```python
from build123d import *

# Parameters (mm, degrees)
SKETCH2_R                = 5
BOSS_EXTRUDE1_DEPTH      = 10
BOSS_EXTRUDE2_DEPTH      = 70
BOSS_EXTRUDE2_DEPTH_BACK = 20
SKETCH2_3_W              = 100
SKETCH2_3_H              = 10
SKETCH3_R                = 5
CUT_EXTRUDE1_DEPTH       = 5
FILLET1_R                = 2


with BuildPart() as part:
    # Sketch2 → Boss-Extrude1 (new body)
    with BuildSketch(Plane(origin=(0, 0, 0), x_dir=(0, 0, -1), z_dir=(1, 0, 0))):
        with BuildLine():
            Line((-8.38684039, 61.382374771), (-45, 5))
            Line((-45, 5), (45, 5))
            Line((45, 5), (8.38684039, 61.382374771))
            ThreePointArc((8.38684039, 61.382374771), (0, 65.936191862), (-8.38684039, 61.382374771))
        make_face()
        with Locations((0, 55.936191862)):
            Circle(SKETCH2_R, mode=Mode.SUBTRACT)
    extrude(amount=BOSS_EXTRUDE1_DEPTH)

    # Sketch2_3 → Boss-Extrude2 (add, two sides: drawn at the far end of the back side and taken through both)
    with BuildSketch(Plane(origin=(0, 0, 0), x_dir=(0, 0, -1), z_dir=(1, 0, 0)).offset(-BOSS_EXTRUDE2_DEPTH_BACK)):
        Rectangle(SKETCH2_3_W, SKETCH2_3_H)
    extrude(amount=BOSS_EXTRUDE2_DEPTH + BOSS_EXTRUDE2_DEPTH_BACK)

    # Sketch3 → Cut-Extrude1 (cut, symmetric)
    with BuildSketch(Plane(origin=(0, 0, 0), x_dir=(1, 0, 0), z_dir=(0, 1, 0))):
        with Locations(Location((60, 40, 0), (0, 0, 270))):
            Circle(SKETCH3_R)
        with Locations(Location((60, -40, 0), (0, 0, 270))):
            Circle(SKETCH3_R)
    extrude(amount=CUT_EXTRUDE1_DEPTH, both=True, mode=Mode.SUBTRACT)

    # Fillet1
    fillet1_edges = [part.edges().sort_by_distance(p)[0] for p in [
        (5, 5, -45),
        (5, 5, 45),
    ]]
    fillet(fillet1_edges, radius=FILLET1_R)


solid = part.part
```
Geometry check sheet. Reference: the model listing, model coordinates, mm. A direction names the side the tool comes from. Round coordinates to 2 decimals unless told otherwise and drop trailing zeros. Order: outer loops, then holes, each group sorted by start corner. A loop starts at its lowest first (then second) coordinate and runs counter-clockwise, first axis right, second up. Notation, with made-up numbers: M 76,-38.75 L 110,-38.75 A23 cw 110,0.25 Z; hole C 73,84.5 d4. An arc over 180 degrees is marked long. Write item = value, one per line.
Q1. Section check B-B (z = 0). Enter the section's corners in (x, y).
Answer block:
outline = M -20,-5 L 70,-5 L 70,5 L 10,5 L 10,50.94 L 0,50.94 L 0,5 L -20,5 Z; M 0,60.94 L 10,60.94 L 10,65.94 L 0,65.94 Z
Q2. Section check C-C (y = 57.5). Enter the section's corners in (x, z).
Answer block:
outline = M 0,-10.91 L 10,-10.91 L 10,-4.75 L 0,-4.75 Z; M 0,4.75 L 10,4.75 L 10,10.91 L 0,10.91 Z
Q3. Scan lines: line 1 (Y direction, x = 5.5, z = 0); line 2 (Z direction, x = 59, y = 1.5); line 3 (Y direction, x = 50, z = -27.5). Record each from-to range of solid material in increasing order.
Answer block:
line_1 = -5 to 50.94, 60.94 to 65.94
line_2 = -50 to -44.9, -35.1 to 35.1, 44.9 to 50
line_3 = -5 to 5
Q4. Section check A-A (x = 60). Enter the section's corners in (y, z).
Answer block:
outline = M -5,-50 L 5,-50 L 5,-45 L -5,-45 Z; M -5,-35 L 5,-35 L 5,35 L -5,35 Z; M -5,45 L 5,45 L 5,50 L -5,50 Z
Q5. Set-up check for faces 4 (the flat face through (0, 29, 1)), 5 (the flat face through (10, 29, 1)), 6 (the flat face through (70, 0, 1)): record each of +Z, -Z, +X, -X, +Y, -Y from which the full face is reachable in a straight line by a thin tool's end or side.
Answer block:
face_4 = +Z, -Z, -X, +Y
face_5 = +Z, -Z, +X, +Y
face_6 = +Z, -Z, +X, +Y, -Y
Q6. Section check D-D (x = 8). Enter the section's corners in (y, z), plus the area to 3 significant figures.
Answer block:
outline = M -5,-50 L 5,-50 L 5,-46.09 A2 cw 5.91,-44.41 L 61.38,-8.39 A10 ccw 61.38,8.39 L 5.91,44.41 A2 cw 5,46.09 L 5,50 L -5,50 Z; hole C 55.94,0 d10
area = 3,990 mm^2
Q7. Release check for a two-part mould opening along Y. For faces 1 (the cylindrical face through (4.93, 65.935, -0.139)), 2 (the flat face through (24, 0, 50)), 3 (the cylindrical face through (4.93, 60.894, 0.651)) record: released by +Y, released by -Y, zero draft, split by the parting line, or undercut.
Answer block:
face_1 = released by +Y
face_2 = zero draft
face_3 = undercut
Q8. Depth check by flat-ended pin: pin 1 Ø10 at (y, z) = (20, 31) entering from -X; pin 2 Ø6 at (x, z) = (13.5, 6) entering from +Y. Enter the tip coordinate at first touch or a pass-through.
Answer block:
pin_1 = 0
pin_2 = 5
